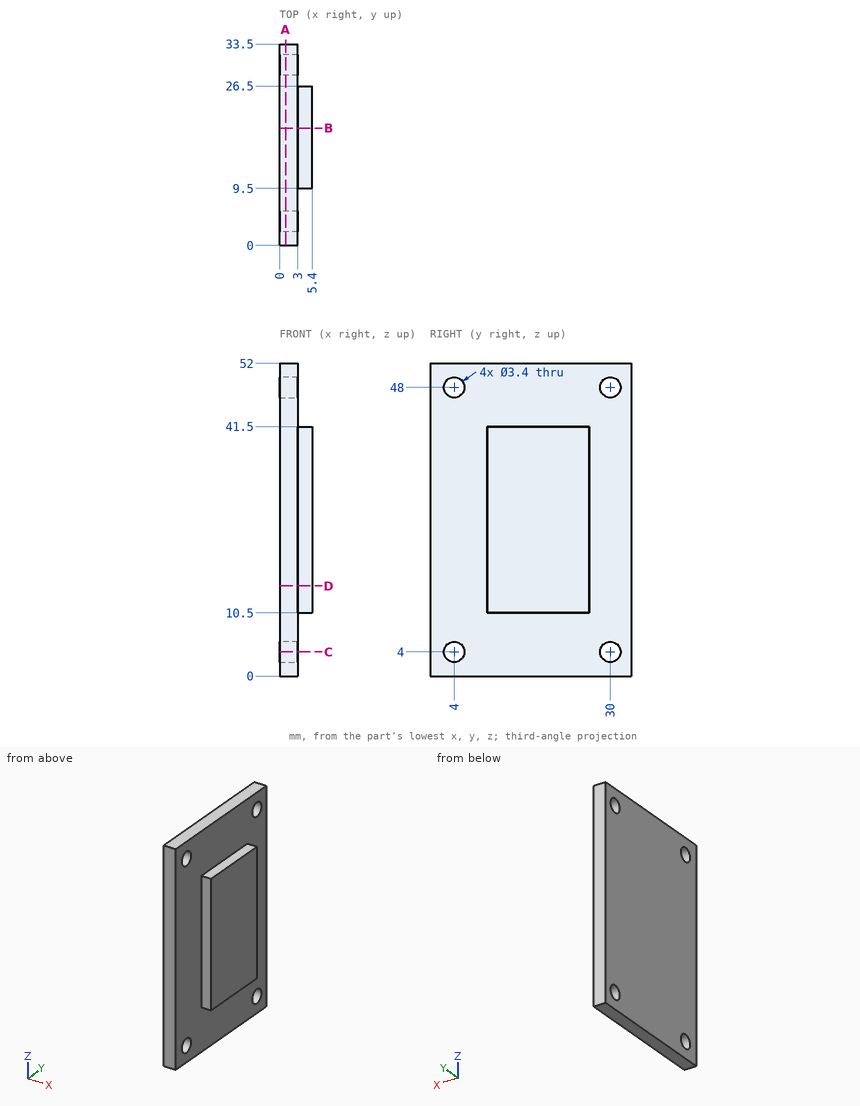
For this review, use the dimensioned drawing (mm, ordinates from the lowest corner) and the shaded views. Coordinates: 2 decimals unless noted, no trailing zeros. Write each loop counter-clockwise with the first axis right and the second up, starting at its lowest first coordinate (ties: lowest second). Pieces come first, ordered by that corner, then holes. Notation, with made-up numbers: (3, 3) - (48, 3) arc R25 cw to (48, 38) - close; hole circle Ø8 at (-7, 76). An arc over 180 degrees is marked (long way). One line per item, written item: value.
1) Add section A-A (x = 1). State the section outline as (y, z) points, plus the area to 3 significant figures.
Answer sheet:
outline: (0, 0) - (33.5, 0) - (33.5, 52) - (0, 52) - close; hole circle Ø3.4 at (4, 4); hole circle Ø3.4 at (4, 48); hole circle Ø3.4 at (30, 4); hole circle Ø3.4 at (30, 48)
area: 1,710 mm2
2) Add section B-B (y = 19.5). State the section outline as (x, z) points, plus the area to 3 significant figures.
Answer sheet:
outline: (0, 0) - (3, 0) - (3, 10.5) - (5.4, 10.5) - (5.4, 41.5) - (3, 41.5) - (3, 52) - (0, 52) - close
area: 230 mm2
3) Add section C-C (z = 4). State the section outline as (x, y) points.
Answer sheet:
outline: (0, 0) - (3, 0) - (3, 2.3) - (0, 2.3) - close; (0, 5.7) - (3, 5.7) - (3, 28.3) - (0, 28.3) - close; (0, 31.7) - (3, 31.7) - (3, 33.5) - (0, 33.5) - close
4) To check wall thickness, follow probe 1 along Y at (x, z) = (1.9, 4); probe 2 along Z at (x, y) = (1.65, 4); probe 3 along Y at (x, z) = (3.95, 28). State the ranges of each line that lie inside material, in increasing order.
Answer sheet:
probe 1: y = 0 to 2.3, 5.7 to 28.3, 31.7 to 33.5
probe 2: z = 0 to 2.3, 5.7 to 46.3, 49.7 to 52
probe 3: y = 9.5 to 26.5
5) Add section D-D (z = 15). State the section outline as (x, y) points, plus the area to 3 significant figures.
Answer sheet:
outline: (0, 0) - (3, 0) - (3, 9.5) - (5.4, 9.5) - (5.4, 26.5) - (3, 26.5) - (3, 33.5) - (0, 33.5) - close
area: 141 mm2
6) Insertion check: pin 1 (2 mm diameter, centred on y = 27.5, z = 42.5, fed in from +X); pin 2 (2.5 mm diameter, centred on x = 4.5, z = 32, fed in from +Y); pin 3 (1.9 mm diameter, centred on x = 4, y = 20, fed in from +Z). Each pin has a flat end and moves straight along its axis. Give the tip position at first contact, or say it passes through.
Answer sheet:
pin 1: stops at x = 3
pin 2: stops at y = 26.5
pin 3: stops at z = 41.5
